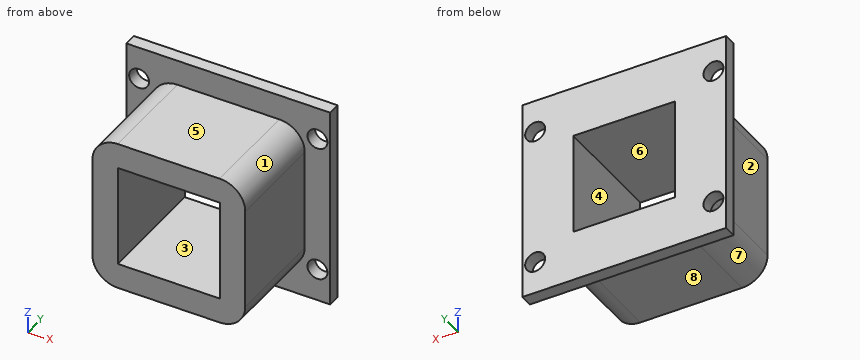
```python
from build123d import *

# Parameters (mm, degrees)
SKETCH1_W           = 50.8
SKETCH1_H           = 50.8
SKETCH1_R           = 2.4892
BOSS_EXTRUDE1_DEPTH = 3.175
BOSS_EXTRUDE2_DEPTH = 25.4
SKETCH2_W           = 25.4
SKETCH2_H           = 25.4
CUT_EXTRUDE1_DEPTH  = 29.575


with BuildPart() as part:
    # Sketch1 → Boss-Extrude1 (new body)
    with BuildSketch(Plane(origin=(0, 0, 0), x_dir=(1, 0, 0), z_dir=(0, 1, 0))):
        Rectangle(SKETCH1_W, SKETCH1_H)
        with Locations((-22.225, 17.2466)):
            Circle(SKETCH1_R, mode=Mode.SUBTRACT)
        with Locations((22.225, 17.2466)):
            Circle(SKETCH1_R, mode=Mode.SUBTRACT)
        with Locations((22.225, -17.2466)):
            Circle(SKETCH1_R, mode=Mode.SUBTRACT)
        with Locations((-22.225, -17.2466)):
            Circle(SKETCH1_R, mode=Mode.SUBTRACT)
    extrude(amount=BOSS_EXTRUDE1_DEPTH)

    # Sketch1<3> → Boss-Extrude2 (add)
    with BuildSketch(Plane(origin=(0, 0, 0), x_dir=(1, 0, 0), z_dir=(0, 1, 0))):
        with BuildLine():
            ThreePointArc((-19.05, -12.7), (-17.190128061, -17.190128061), (-12.7, -19.05))
            Line((-12.7, -19.05), (12.7, -19.05))
            ThreePointArc((12.7, -19.05), (17.190128061, -17.190128061), (19.05, -12.7))
            Line((19.05, -12.7), (19.05, 12.7))
            ThreePointArc((19.05, 12.7), (17.190128061, 17.190128061), (12.7, 19.05))
            Line((12.7, 19.05), (-12.7, 19.05))
            ThreePointArc((-12.7, 19.05), (-17.190128061, 17.190128061), (-19.05, 12.7))
            Line((-19.05, 12.7), (-19.05, -12.7))
        make_face()
    extrude(amount=-BOSS_EXTRUDE2_DEPTH)

    # Sketch2 → Cut-Extrude1 (cut, through all)
    with BuildSketch(Plane(origin=(0, 3.175, 0), x_dir=(1, 0, 0), z_dir=(0, 1, 0))):
        Rectangle(SKETCH2_W, SKETCH2_H)
    extrude(amount=-CUT_EXTRUDE1_DEPTH, mode=Mode.SUBTRACT)


solid = part.part
```
Source: CAD feature listing. Evaluate the final solid. Frame: model axes, mm. Face numbers are marked on the shaded views. A direction names the side the tool comes from. Coordinates: 2 decimals unless noted, no trailing zeros. Loops run counter-clockwise (first coordinate to the right, second up) from the corner with the lowest first, then second, coordinate; pieces in that order, holes last. Notation, with made-up numbers: M 38,61.5 L 83,61.5 A18 ccw 83,79.5 Z; hole C 55,-3 d1. An arc over 180 degrees is marked long. Put each result on its own line as item: value. Start each with the question number.
1) Cut plane C-C on y = -9. Return the cut outline in (x, z), then the cut area to 3 significant figures.
2) Cut plane A-A on z = -11. Return the cut outline in (x, y) (3 decimals), then the cut area to 3 significant figures.
3) Reachability of the marked faces 5, 6, 7 and 8 from +Z, -Z, +X, -X, +Y, -Y: full face, straight path, thin tool, end or side. Return the list, or none.
4) Cut plane D-D on x = 20.5. Return the cut outline in (y, z) (3 decimals).
5) Contact query for flat-ended pins moving along their axis: pin 1 Ø2 at (y, z) = (-15.5, -9) entering from -X; pin 2 Ø5.5 at (x, z) = (22.22, -17.25) entering from -Y; pin 3 Ø12.5 at (x, y) = (2, -11) entering from -Z; pin 4 Ø4 at (x, z) = (22.22, 17.25) entering from -Y. Output: stop coordinate, or through.
6) Pull-direction query (Z, two-part tool) for the marked faces 1, 2, 3 and 4; classes: pulls with the +Z half, pulls with the -Z half, needs draft (parallel to the pull), parting line crosses it, or undercut.
7) Cut plane B-B on x = 6.5. Return the cut outline in (y, z) (3 decimals), then the cut area to 3 significant figures.
8) Ray query, L1, parallel to Z at x = -2.5, y = -10.5; L2, parallel to Y at x = -23, z = 9 (3 decimals). Return the intervals inside material, ascending. Write a range as from..to.
The answers:
1. outline: M -19.05,-12.7 A6.35 ccw -12.7,-19.05 L 12.7,-19.05 A6.35 ccw 19.05,-12.7 L 19.05,12.7 A6.35 ccw 12.7,19.05 L -12.7,19.05 A6.35 ccw -19.05,12.7 Z; hole M -12.7,-12.7 L 12.7,-12.7 L 12.7,12.7 L -12.7,12.7 Z
1. area: 772 mm²
2. outline: M -25.4,0 L -19.05,0 L -19.05,-25.4 L -12.7,-25.4 L -12.7,3.175 L -25.4,3.175 Z; M 12.7,-25.4 L 19.05,-25.4 L 19.05,0 L 25.4,0 L 25.4,3.175 L 12.7,3.175 Z
2. area: 403 mm²
3. face 5: +Z, +X, -X, -Y
3. face 6: +Y, -Y
3. face 7: -Z, -X, -Y
3. face 8: -Z, +X, -X, -Y
4. outline: M 0,-25.4 L 3.175,-25.4 L 3.175,-19.041 L 0,-19.041 Z; M 0,-15.452 L 3.175,-15.452 L 3.175,15.452 L 0,15.452 Z; M 0,19.041 L 3.175,19.041 L 3.175,25.4 L 0,25.4 Z
5. pin 1: stops at x = -19.05
5. pin 2: stops at y = 0
5. pin 3: stops at z = -19.05
5. pin 4: passes through
6. face 1: pulls with the +Z half
6. face 2: needs draft
6. face 3: undercut
6. face 4: undercut
7. outline: M -25.4,-19.05 L 0,-19.05 L 0,-25.4 L 3.175,-25.4 L 3.175,-12.7 L -25.4,-12.7 Z; M -25.4,12.7 L 3.175,12.7 L 3.175,25.4 L 0,25.4 L 0,19.05 L -25.4,19.05 Z
7. area: 403 mm²
8. L1: z = -19.05..-12.7, 12.7..19.05
8. L2: y = 0..3.175
